Part model, mm, in its own coordinate system. Face numbers are marked on the shaded views. A direction names the side the tool comes from. Round coordinates to 2 decimals unless told otherwise and drop trailing zeros. Loops run counter-clockwise (first coordinate to the right, second up) from the corner with the lowest first, then second, coordinate; pieces in that order, holes last. Notation, with made-up numbers: (-36.75, -0.75) -> (-15.75, -0.75) arc R35 ccw to (-15.75, 33.25) -> close; hole circle Ø2 at (-31, 77.25). An arc over 180 degrees is marked (long way). Answer as a JSON object with one key per item and string values. Group by question number.
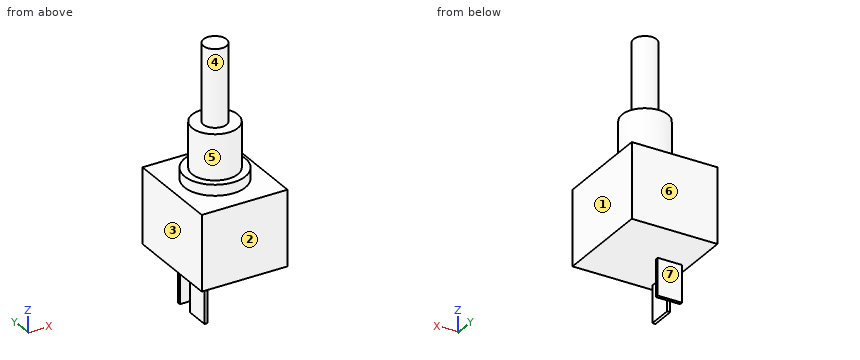
from build123d import *

# Parameters (mm, degrees)
F0_W     = 22.25
F0_H     = 25.4
F1_DEPTH = 19.5
F2_R     = 7.9
F2_R_2   = 5.95
F3_DEPTH = 2.8
F4_R     = 5.95
F5_DEPTH = 11.75
F6_R     = 3
F7_DEPTH = 20
F8_W     = 0.8
F8_H     = 6.3
F8_W_2   = 6.3
F8_H_2   = 0.8
F9_DEPTH = 9.6


with BuildPart() as f1:
    # F0 (on Top) → F1 (new body)
    with BuildSketch(Plane.XY):
        Rectangle(F0_W, F0_H)
    extrude(amount=F1_DEPTH)

    # F2 (on face) → F3 (join)
    with BuildSketch(Plane.XY.offset(19.5)):
        Circle(F2_R)
        Circle(F2_R_2, mode=Mode.SUBTRACT)
        Circle(F2_R_2)
    extrude(amount=F3_DEPTH)

    # F4 (on face) → F5 (join)
    with BuildSketch(Plane.XY.offset(22.3)):
        Circle(F4_R)
    extrude(amount=F5_DEPTH)

    # F6 (on face) → F7 (join)
    with BuildSketch(Plane.XY.offset(34.05)):
        Circle(F6_R)
    extrude(amount=F7_DEPTH)

    # F8 (on face) → F9 (join)
    with BuildSketch(Plane(origin=(0, 0, 0), x_dir=(1, 0, 0), z_dir=(0, 0, -1))):
        with Locations((-8.925, 7.75)):
            Rectangle(F8_W, F8_H)
        with Locations((-6.175, -0.05)):
            Rectangle(F8_W_2, F8_H_2)
    extrude(amount=F9_DEPTH)


solid = f1.part
Item 1: Drill centre lines: line 1 (Z direction, x = 7.5, y = -9); line 2 (Z direction, x = 1.25, y = -2); line 3 (Y direction, x = -4.5, z = 23.5). Where is each one in solid material? Low to high.
Item 2: Band-saw the part on A-A, the plane x = 0. List the corners of the cut face in (y, z).
Item 3: Which spindle directions (+Z, -Z, +X, -X, +Y, -Y) get a long thin tool onto all of the face, cutting with end or side? Do the marked faces 5, 6 and 7. Say none if no direction does.
Item 4: Two-plate mould, pull along X, no slides. Class the marked faces 1, 2, 3 and 4: pulls with the +X half, pulls with the -X half, needs draft (parallel to the pull), parting line crosses it, or undercut.
Item 5: Band-saw the part on B-B, the plane x = -4.5. List the corners of the cut face in (y, z).
Item 6: Drop flat-ended pins along their axis: pin 1 Ø10 at (x, y) = (-4, 8.5) entering from -Z; pin 2 Ø2 at (x, z) = (-5.5, 28) entering from +Y; pin 3 Ø8 at (x, z) = (6.5, 27.5) entering from -Y; pin 4 Ø8 at (x, y) = (-1, 3.5) entering from +Z. Give the stop position or say it passes through.
Entries:
{
 "1": {"line 1": "0 to 19.5", "line 2": "0 to 54.05", "line 3": "-3.89 to 3.89"},
 "2": {"outline": "(-12.7, 0) -> (12.7, 0) -> (12.7, 19.5) -> (7.9, 19.5) -> (7.9, 22.3) -> (5.95, 22.3) -> (5.95, 34.05) -> (3, 34.05) -> (3, 54.05) -> (-3, 54.05) -> (-3, 34.05) -> (-5.95, 34.05) -> (-5.95, 22.3) -> (-7.9, 22.3) -> (-7.9, 19.5) -> (-12.7, 19.5) -> close"},
 "3": {"face 5": "+Z", "face 6": "+Z, -Z, +X, -X, +Y", "face 7": "-Z, +X, -X, +Y"},
 "4": {"face 1": "pulls with the +X half", "face 2": "needs draft", "face 3": "pulls with the -X half", "face 4": "parting line crosses it"},
 "5": {"outline": "(-12.7, 0) -> (-0.35, 0) -> (-0.35, -9.6) -> (0.45, -9.6) -> (0.45, 0) -> (12.7, 0) -> (12.7, 19.5) -> (6.49, 19.5) -> (6.49, 22.3) -> (3.89, 22.3) -> (3.89, 34.05) -> (-3.89, 34.05) -> (-3.89, 22.3) -> (-6.49, 22.3) -> (-6.49, 19.5) -> (-12.7, 19.5) -> close"},
 "6": {"pin 1": "z = 0", "pin 2": "y = 3.89", "pin 3": "y = -5.4", "pin 4": "z = 54.05"}
}
